```python
from build123d import *

# Parameters (mm, degrees)
F0_W     = 85.474864
F0_H     = 83.643266
F2_DEPTH = 25.4
F1_R     = 21.045821
F3_DEPTH = 44.958
F5_DEPTH = 32.766


with BuildPart() as f2:
    # F0 (on Top) → F2 (new body)
    with BuildSketch(Plane.XY):
        Rectangle(F0_W, F0_H)
    extrude(amount=F2_DEPTH)

    # F1 (on face) → F3 (join)
    with BuildSketch(Plane.XY):
        Circle(F1_R)
    extrude(amount=F3_DEPTH)

    # F4 (on Right) → F5 (cut, symmetric)
    with BuildSketch(Plane.YZ):
        Polygon((25.421897, 37.048966), (25.421897, 48.478965), (-27.195517, 49.070172), (-27.195517, 28.37793), align=None)
    extrude(amount=F5_DEPTH, both=True, mode=Mode.SUBTRACT)


solid = f2.part
```
Could you check a few things on this model? Use its own coordinates, in mm. A direction names the side the tool comes from. Round coordinates to 2 decimals unless told otherwise and drop trailing zeros. Order: outer loops, then holes, each group sorted by start corner. A loop starts at its lowest first (then second) coordinate and runs counter-clockwise, first axis right, second up. Notation, with made-up numbers: M -32.5,-6.5 L 17.5,-6.5 A25 ccw 17.5,23.5 Z; hole C 13.25,-22.75 d1. An arc over 180 degrees is marked long. One line per question, with ' | ' between items. Start each with the question number.
(1) Suppose I cut it at C-C on y = -27. List the corners of the cut face in (x, z) for me.
(2) Suppose I cut it at B-B on y = -4. List the corners of the cut face in (x, z) for me.
(3) For P1, Ø4, axis at x = 19.5, z = 27, coming from the +Y side; P2, Ø3, axis at x = 7, y = -14, coming from the +Z side, each with a flat end and sliding along its axis, tell me the tip position at first contact or that it passes through.
(4) Please list where these lines run through material, in increasing order: line 1 along Z through (x, y) = (-22, 7.5); line 2 along X through (y, z) = (-8, 26); line 3 along X through (y, z) = (19.5, 33).
(5) For faces 1 (the face through (-10, 19, 25.4)), 2 (the face through (42.737, -1, 13)), which set-ups out of +Z, -Z, +X, -X, +Y, -Y let a thin tool reach every point of the face, with its end or its side?
(6) Suppose I cut it at D-D on x = 37.5. List the corners of the cut face in (y, z) for me, then the cut area to 3 significant figures.
(7) Suppose I cut it at A-A on x = 0. List the corners of the cut face in (y, z) for me, then the cut area to 3 significant figures.
Geometry results:
1) outline: M -42.74,0 L 42.74,0 L 42.74,25.4 L -42.74,25.4 Z
2) outline: M -42.74,0 L 42.74,0 L 42.74,25.4 L 20.66,25.4 L 20.66,32.2 L -20.66,32.2 L -20.66,25.4 L -42.74,25.4 Z
3) P1: y = 41.82 | P2: z = 30.8
4) line 1: 0 to 25.4 | line 2: -19.47 to 19.47 | line 3: -7.92 to 7.92
5) face 1: +Z | face 2: +Z, -Z, +X, +Y, -Y
6) outline: M -41.82,0 L 41.82,0 L 41.82,25.4 L -41.82,25.4 Z | area: 2,120 mm²
7) outline: M -41.82,0 L 41.82,0 L 41.82,25.4 L 21.05,25.4 L 21.05,36.33 L -21.05,29.39 L -21.05,25.4 L -41.82,25.4 Z | area: 2,440 mm²
